Geometry check sheet. Reference: the model listing, model coordinates, mm. Round coordinates to 2 decimals unless told otherwise and drop trailing zeros. Order: outer loops, then holes, each group sorted by start corner. A loop starts at its lowest first (then second) coordinate and runs counter-clockwise, first axis right, second up.
```python
from build123d import *

# Parameters (mm, degrees)
F0_W     = 1180
F0_H     = 880
F1_DEPTH = 35
F2_R     = 3
F3_DEPTH = 20
F5_W     = 1120
F5_H     = 820
F6_DEPTH = 10


with BuildPart() as f1:
    # F0 (on Top) → F1 (new body)
    with BuildSketch(Plane.XY):
        with Locations((-536.928684, 412.954066)):
            Rectangle(F0_W, F0_H)
    extrude(amount=F1_DEPTH)

    # F2 (on face) → F3 (cut)
    with BuildSketch(Plane(origin=(0, 0, 0), x_dir=(1, 0, 0), z_dir=(0, 0, -1))):
        with Locations((-1016.928684, -82.954066)):
            Circle(F2_R)
    extrude(amount=-F3_DEPTH, mode=Mode.SUBTRACT)

    # F5 (on face) → F6 (cut)
    with BuildSketch(Plane.XY.offset(35)):
        with Locations((-536.928684, 412.954066)):
            Rectangle(F5_W, F5_H)
    extrude(amount=-F6_DEPTH, mode=Mode.SUBTRACT)


solid = f1.part
```
(1) Sectioned sample at B-B, the plane y = 670. Record the cut outline in (x, z).
Returned:
outline: (-1126.93, 0) - (53.07, 0) - (53.07, 35) - (23.07, 35) - (23.07, 25) - (-1096.93, 25) - (-1096.93, 35) - (-1126.93, 35) - close
(2) Depth check by flat-ended pin: P1, Ø3, axis at x = -1016, y = 83.5, coming from the -Z side; P2, Ø1, axis at x = -536, y = 516.5, coming from the +Z side. Enter the tip coordinate at first touch or a pass-through.
Returned:
P1: stops at z = 20
P2: stops at z = 25
(3) Draft check along X on faces 1 (the flat face through (-545, 419, 25)), 2 (the flat face through (-1126.929, 407, 17)), 3 (the flat face through (-545, 852.954, 17)). Enter one of: released by +X, released by -X, zero draft, split by the parting line, or undercut.
Returned:
face 1: undercut
face 2: released by -X
face 3: zero draft
(4) Sectioned sample at A-A, the plane x = -47.5. Record the cut outline in (y, z).
Returned:
outline: (-27.05, 0) - (852.95, 0) - (852.95, 35) - (822.95, 35) - (822.95, 25) - (2.95, 25) - (2.95, 35) - (-27.05, 35) - close
(5) Material ranges on line 1 (Y direction, x = -889, z = 26); line 2 (X direction, y = 167.5, z = 28); line 3 (Z direction, x = -761, y = 378.5), recorded low to high.
Returned:
line 1: y = -27.05 to 2.95, 822.95 to 852.95
line 2: x = -1126.93 to -1096.93, 23.07 to 53.07
line 3: z = 0 to 25
